from build123d import *

# Parameters (mm, degrees)
F0_W     = 101.6
F0_H     = 50.8
F0_R     = 1.905
F1_DEPTH = 3.81
F3_R     = 1.905
F4_DEPTH = 12.7
F6_R     = 1.905
F7_DEPTH = 12.7


with BuildPart() as f1:
    # F0 (on Front) → F1 (new body, symmetric)
    with BuildSketch(Plane.XZ):
        Rectangle(F0_W, F0_H)
        with Locations((-38.1, -22.225)):
            Circle(F0_R, mode=Mode.SUBTRACT)
        with Locations((-19.05, -22.225)):
            Circle(F0_R, mode=Mode.SUBTRACT)
        with Locations((0, -22.225)):
            Circle(F0_R, mode=Mode.SUBTRACT)
        with Locations((19.05, -22.225)):
            Circle(F0_R, mode=Mode.SUBTRACT)
        with Locations((38.1, -22.225)):
            Circle(F0_R, mode=Mode.SUBTRACT)
        with Locations((-38.1, 22.225)):
            Circle(F0_R, mode=Mode.SUBTRACT)
        with Locations((-19.05, 22.225)):
            Circle(F0_R, mode=Mode.SUBTRACT)
        with Locations((0, 22.225)):
            Circle(F0_R, mode=Mode.SUBTRACT)
        with Locations((19.05, 22.225)):
            Circle(F0_R, mode=Mode.SUBTRACT)
        with Locations((38.1, 22.225)):
            Circle(F0_R, mode=Mode.SUBTRACT)
    extrude(amount=F1_DEPTH, both=True)

    # F3 (on offset) → F4 (cut)
    with BuildSketch(Plane.YZ.offset(50.8)):
        Circle(F3_R)
    extrude(amount=-F4_DEPTH, mode=Mode.SUBTRACT)

    # F6 (on offset) → F7 (cut)
    with BuildSketch(Plane(origin=(-50.8, 0, 0), x_dir=(0, -1, 0), z_dir=(-1, 0, 0))):
        Circle(F6_R)
    extrude(amount=-F7_DEPTH, mode=Mode.SUBTRACT)


solid = f1.part
For this review, take the finished solid that the model builds, in its own axes (mm). A direction names the side the tool comes from. Round coordinates to 2 decimals unless told otherwise and drop trailing zeros. Order: outer loops, then holes, each group sorted by start corner. A loop starts at its lowest first (then second) coordinate and runs counter-clockwise, first axis right, second up. Notation, with made-up numbers: M 14.5,73 L 63.5,73 A26 ccw 63.5,95 Z; hole C 70.5,-17.5 d1. An arc over 180 degrees is marked long. Use a Markdown table: item, result. Add a question column.
Item 1: To check wall thickness, follow line 1 along X through (y, z) = (-3, 22.5); line 2 along Z through (x, y) = (-19.05, -2); line 3 along X through (y, z) = (2.75, -21). State the ranges of each line that lie inside material, in increasing order.
Item 2: Insertion check: pin 1 (4 mm diameter, centred on y = -0.5, z = -0.5, fed in from +X); pin 2 (2.5 mm diameter, centred on y = 0, z = 0, fed in from -X); pin 3 (3.5 mm diameter, centred on y = 0, z = 0, fed in from +X). Each pin has a flat end and moves straight along its axis. Give the tip position at first contact, or say it passes through.
Item 3: Add section D-D, the plane x = -42.5. Give the boundary of the cut face in (y, z) (3 decimals), then the cut area to 3 significant figures.
Item 4: Add section B-B, the plane y = -0.75. State how many separate pieces and enclosed holes the cut face has, then the cut area to 3 significant figures.
Item 5: Add section A-A, the plane x = 19.05. Give the boundary of the cut face in (y, z).
Item 6: Tool access review of faces 1 (the flat face through (-50.8, -3, 0)), 2 (the flat face through (-38.1, 0, 0)): name each direction out of +Z, -Z, +X, -X, +Y, -Y from which nothing blocks a thin tool from reaching the whole face with its end or side.
Item 7: Add section C-C, the plane z = 0. Give the boundary of the cut face in (x, y) (3 decimals).
Item 8: Mouldability with a two-part tool opening along Z and no side actions: class faces 3 (the flat face through (-1, 3.81, 0)), 4 (the flat face through (38.1, 0, 0)), 5 (the flat face through (-1, 0, 25.4)) as released by +Z, released by -Z, zero draft, split by the parting line, or undercut.
Geometry results:
| question | item | result |
|---|---|---|
| 1 | line 1 | x = -50.8 to -39.99, -36.21 to -20.94, -17.16 to -1.89, 1.89 to 17.16, 20.94 to 36.21, 39.99 to 50.8 |
| 1 | line 2 | z = -25.4 to -24.13, -20.32 to 20.32, 24.13 to 25.4 |
| 1 | line 3 | x = -50.8 to -39.56, -36.64 to -20.51, -17.59 to -1.46, 1.46 to 17.59, 20.51 to 36.64, 39.56 to 50.8 |
| 2 | pin 1 | stops at x = 50.8 |
| 2 | pin 2 | stops at x = -38.1 |
| 2 | pin 3 | stops at x = 38.1 |
| 3 | outline | M -3.81,-25.4 L 3.81,-25.4 L 3.81,25.4 L -3.81,25.4 Z; hole C 0,0 d3.81 |
| 3 | area | 376 mm² |
| 4 | separate pieces | 1 |
| 4 | enclosed holes | 10 |
| 4 | area | 4,960 mm² |
| 5 | outline | M -3.81,-25.4 L 3.81,-25.4 L 3.81,-24.13 L -3.81,-24.13 Z; M -3.81,-20.32 L 3.81,-20.32 L 3.81,20.32 L -3.81,20.32 Z; M -3.81,24.13 L 3.81,24.13 L 3.81,25.4 L -3.81,25.4 Z |
| 6 | face 1 | +Z, -Z, -X, +Y, -Y |
| 6 | face 2 | -X |
| 7 | outline | M -50.8,-3.81 L 50.8,-3.81 L 50.8,-1.905 L 38.1,-1.905 L 38.1,1.905 L 50.8,1.905 L 50.8,3.81 L -50.8,3.81 L -50.8,1.905 L -38.1,1.905 L -38.1,-1.905 L -50.8,-1.905 Z |
| 8 | face 3 | zero draft |
| 8 | face 4 | undercut |
| 8 | face 5 | released by +Z |
